Source: CAD feature listing. Evaluate the final solid. Frame: model axes, mm. Face numbers are marked on the shaded views. A direction names the side the tool comes from. Give positions to 0.01 mm unless a question says otherwise; leave off trailing zeros. Loops run counter-clockwise (first coordinate to the right, second up) from the corner with the lowest first, then second, coordinate; pieces in that order, holes last. Notation, with made-up numbers: M 70,-40 L 128,-40 A15 cw 128,-25 Z; hole C 0.25,17.25 d4. An arc over 180 degrees is marked long. Answer in a Markdown table with one row per item.
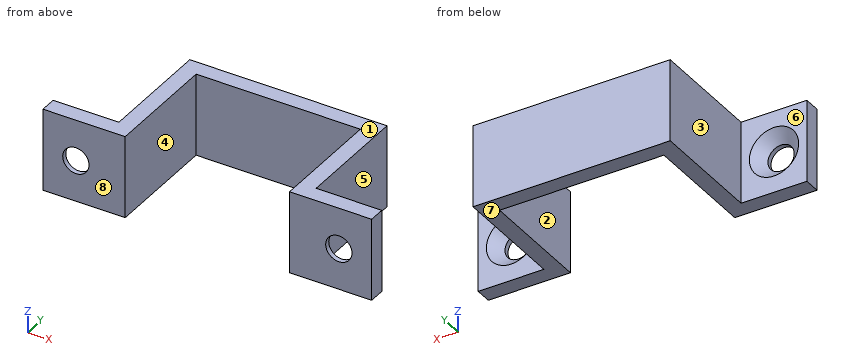
Autodesk Inventor part; units mm, degrees
ref_plane "YZ Plane" through (0, 0, 0) normal (1, 0, 0) x (0, 1, 0)
ref_plane "XZ Plane" through (0, 0, 0) normal (0, 1, 0) x (-1, 0, 0)
ref_plane "XY Plane" through (0, 0, 0) normal (0, 0, 1) x (1, 0, 0)
sketch "Sketch1" plane through (0, 0, 0) normal (0, 0, 1) x (1, 0, 0)
  line L0 (-10, 0) -> (10, 0) construction
  line L1 (10, 0) -> (10, 14)
  line L2 (10, 14) -> (-10, 14)
  line L3 (-10, 14) -> (-10, 0)
  line L4 (-12, -8.7582) -> (12, -8.7582) construction
  line L5 (12, -8.7582) -> (12, 2) construction
  line L6 (12, 16) -> (-12, 16)
  line L7 (-12, 16) -> (-12, 2)
  line L8 (-10, 0) -> (-20, 0)
  line L9 (-20, 0) -> (-20, 2)
  line L10 (-20, 2) -> (-12, 2)
  line L11 (-12, 2) -> (-12, -8.7582) construction
  line L12 (0, 16) -> (0, -8.7582)
  line L13 (10, 0) -> (20, 0)
  line L14 (20, 0) -> (20, 2)
  line L15 (20, 2) -> (12, 2)
  line L16 (12, 2) -> (12, 16)
  point P0 (0, 0)
  point P1 (0, 0)
  dimension "d0" = 14
  dimension "d1" = 20
  dimension "d2" = 2
  dimension "d3" = 2
  dimension "d4" = 10
  dimension "d5" = 2
  dimension "d6" = 2
extrude "Extrusion1" add sketch "Sketch1" along normal blind 10
sketch "Sketch2" plane through (-20, 2, 0) normal (0, 1, 0) x (1, 0, 0)
  line L0 (8, 0) -> (0, 0) construction
  line L1 (0, 0) -> (0, -10) construction
  line L2 (8, -10) -> (0, -10) construction
  line L3 (8, 0) -> (8, -10) construction
  line L4 (40, 0) -> (32, 0) construction
  line L5 (32, 0) -> (32, -10) construction
  line L6 (40, -10) -> (32, -10) construction
  line L7 (40, 0) -> (40, -10) construction
  line L8 (8, -10) -> (0, 0) construction
  line L9 (0, -10) -> (8, 0) construction
  line L10 (40, -10) -> (32, 0) construction
  line L11 (32, -10) -> (40, 0) construction
  point P0 (20, 0)
  point P1 (4, -5)
  point P2 (36, -5)
hole "Hole1" at (-16, 2, 5) at (16, 2, 5) direction (0, -1, 0) diameter 3.2 end through all countersink diameter 6 countersink angle 90
properties part number "switchHolder"
Q1. Section query A-A (z = 5). Output: boundary loops of the cut face in (x, y), plus the area to 3 significant figures.
Values follow:
| item | result |
|---|---|
| outline | M -20,0 L -17.6,0 L -17.6,0.6 L -19,2 L -20,2 Z; M -14.4,0 L -10,0 L -10,14 L 10,14 L 10,0 L 14.4,0 L 14.4,0.6 L 13,2 L 12,2 L 12,16 L -12,16 L -12,2 L -13,2 L -14.4,0.6 Z; M 17.6,0 L 20,0 L 20,2 L 19,2 L 17.6,0.6 Z |
| area | 119 mm^2 |
Q2. Section query B-B (x = -16). Output: boundary loops of the cut face in (y, z).
Values follow:
| item | result |
|---|---|
| outline | M 0,0 L 2,0 L 2,2 L 0.6,3.4 L 0,3.4 Z; M 0,6.6 L 0.6,6.6 L 2,8 L 2,10 L 0,10 Z |
Q3. Section query D-D (z = 9.25). Output: boundary loops of the cut face in (x, y), plus the area to 3 significant figures.
Values follow:
| item | result |
|---|---|
| outline | M -20,0 L -10,0 L -10,14 L 10,14 L 10,0 L 20,0 L 20,2 L 12,2 L 12,16 L -12,16 L -12,2 L -20,2 Z |
| area | 136 mm^2 |
Q4. Section query C-C (y = 9). Output: boundary loops of the cut face in (x, z), plus the area to 3 significant figures.
Values follow:
| item | result |
|---|---|
| outline | M -12,0 L -10,0 L -10,10 L -12,10 Z; M 10,0 L 12,0 L 12,10 L 10,10 Z |
| area | 40.0 mm^2 |
Q5. Mould query, pull axis X, two halves, no side actions, for the marked faces 1, 2 and 3. Classes: +X half, -X half, draft (parallel to the pull), parting line (faces both ways), or undercut.
Values follow:
| item | result |
|---|---|
| face 1 | draft |
| face 2 | undercut |
| face 3 | -X half |
Q6. Contact query for flat-ended pins moving along their axis: pin 1 Ø1 at (y, z) = (8, 4) entering from +X; pin 2 Ø5 at (y, z) = (11.5, 5) entering from -X. Output: stop coordinate, or through.
Values follow:
| item | result |
|---|---|
| pin 1 | x = 12 |
| pin 2 | x = -12 |
Q7. Reachability of the marked faces 4, 5, 6, 7 and 8 from +Z, -Z, +X, -X, +Y, -Y: full face, straight path, thin tool, end or side. Return the list, or none.
Values follow:
| item | result |
|---|---|
| face 4 | +Z, -Z, -Y |
| face 5 | +Z, -Z, +X, +Y |
| face 6 | +Z, -Z, -X, +Y |
| face 7 | -Z, +X, -X, +Y, -Y |
| face 8 | +Z, -Z, +X, -X, -Y |
Q8. Ray query, probe 1 along X at (y, z) = (0.5, 5); probe 2 along X at (y, z) = (13, 6); probe 3 along Z at (x, y) = (16, 0.35). Return the intervals inside material, ascending. Write a range as from..to.
Values follow:
| item | result |
|---|---|
| probe 1 | -20..-17.6, -14.4..-10, 10..14.4, 17.6..20 |
| probe 2 | -12..-10, 10..12 |
| probe 3 | 0..3.4, 6.6..10 |
